Can you work these out from the model? Positions are in its coordinate system, mm. A direction names the side the tool comes from. Give positions to 0.01 mm unless a question says otherwise; leave off trailing zeros. Order: outer loops, then holes, each group sorted by start corner. A loop starts at its lowest first (then second) coordinate and runs counter-clockwise, first axis right, second up. Notation, with made-up numbers: M -17.5,66.25 L 29.5,66.25 A12 cw 29.5,73.25 Z; hole C 52.5,13 d11. An arc over 180 degrees is marked long. One line per question, with ' | ' between items. Start each with the question number.
1) For faces 1 (the flat face through (-17, 0, 39)), 2 (the flat face through (39.498, -13, 50)), 3 (the flat face through (28, -13, 61.81)), 4 (the flat face through (0, -13, 18)), which set-ups out of +Z, -Z, +X, -X, +Y, -Y let a thin tool reach every point of the face, with its end or its side?
2) Please list where these lines run through material, in increasing order: line 1 along Z through (x, y) = (37.5, -9.5); line 2 along Z through (x, y) = (69.5, -5) (3 decimals); line 3 along X through (y, z) = (-22, 63). Write a range as [from, to].
3) Thinking about a two-plate mould opening in X: for faces 5 (the flat face through (28, -13, 52.4)), 6 (the flat face through (39.498, -13, 69)), 7 (the flat face through (65, -13, 47.625)), 8 (the cylindrical face through (4.72, -12.52, 47.83)), which applies, +X half, -X half, draft (parallel to the pull), parting line (faces both ways), or undercut?
4) If we section it at B-B, the plane x = 47.5: Please give me the cut outline in (y, z) (3 decimals), plus the area to 3 significant figures.
5) If we section it at A-A, the plane z = 7.5: Please give me the cut outline in (x, y).
6) I'm going to push flat-ended pins straight in: pin 1 Ø1 at (x, y) = (-1.5, -21.5) entering from +Z; pin 2 Ø7 at (x, y) = (33.5, -16) entering from +Z; pin 3 Ø4.5 at (y, z) = (-9, 67) entering from -X; pin 4 Ø12 at (x, y) = (-12, -9.5) entering from -Z. Where does each tip first touch, or does it pass through?
```python
from build123d import *

# Parameters (mm, degrees)
F1_DEPTH = 25.4


with BuildPart() as f1:
    # F0 (on Front) → F1 (new body)
    with BuildSketch(Plane.XZ):
        Polygon((-82.55, 0), (0, 0), (0, 19.05), (-9.4102, 19.05), (-82.55, 19.05), align=None)
        with BuildLine():
            Line((-9.4102, 19.05), (0, 19.05))
            Line((0, 19.05), (0, 36.535349))
            ThreePointArc((0, 36.535349), (4.852166, 47.959566), (16.442551, 52.4002))
            Line((16.442551, 52.4002), (39.498304, 52.4002))
            Line((39.498304, 52.4002), (39.498304, 61.8104))
            Line((39.498304, 61.8104), (16.591319, 61.8104))
            ThreePointArc((16.591319, 61.8104), (14.455766, 61.780687), (12.330339, 61.570857))
            add(Edge.make_bspline(
                [(10.443617, 61.230316), (11.07103, 61.345589), (11.699943, 61.459099), (12.330339, 61.570857)],
                knots=[102.267957, 102.267957, 102.267957, 102.267957, 103.972602, 103.972602, 103.972602, 103.972602], degree=3))
            ThreePointArc((10.443617, 61.230316), (-3.83128, 52.37845), (-9.4102, 36.535349))
            Line((-9.4102, 36.535349), (-9.4102, 19.05))
        make_face()
        with BuildLine():
            add(Edge.make_bspline(
                [(-82.55, 19.05), (-59.439801, 41.052572), (-27.197229, 54.314634), (10.443617, 61.230316)],
                knots=[0, 0, 0, 0, 102.267957, 102.267957, 102.267957, 102.267957], degree=3))
            Line((-82.55, 19.05), (-9.4102, 19.05))
            Line((-9.4102, 19.05), (-9.4102, 36.535349))
            ThreePointArc((-9.4102, 36.535349), (-3.83128, 52.37845), (10.443617, 61.230316))
        make_face()
        with BuildLine():
            ThreePointArc((12.330339, 61.570857), (11.383749, 61.418475), (10.443617, 61.230316))
            add(Edge.make_bspline(
                [(10.443617, 61.230316), (11.07103, 61.345589), (11.699943, 61.459099), (12.330339, 61.570857)],
                knots=[102.267957, 102.267957, 102.267957, 102.267957, 103.972602, 103.972602, 103.972602, 103.972602], degree=3))
        make_face()
        Polygon((39.498304, 61.8104), (39.498304, 52.4002), (39.498304, 47.625), (90.298304, 47.625), (90.298304, 76.2), (39.498304, 76.2), align=None)
    extrude(amount=F1_DEPTH)


solid = f1.part
```
Results found:
1) face 1: +Z, -Z, +X, -X, +Y | face 2: -Z, +Y, -Y | face 3: +Z, -X, +Y, -Y | face 4: -Z, +X, +Y, -Y
2) line 1: z = [52.4, 61.81] | line 2: z = [47.625, 76.2] | line 3: x = [39.5, 90.3]
3) face 5: undercut | face 6: -X half | face 7: draft | face 8: undercut
4) outline: M -25.4,47.625 L 0,47.625 L 0,76.2 L -25.4,76.2 Z | area: 726 mm²
5) outline: M -82.55,-25.4 L 0,-25.4 L 0,0 L -82.55,0 Z
6) pin 1: stops at z = 58.89 | pin 2: stops at z = 61.81 | pin 3: stops at x = 39.5 | pin 4: stops at z = 0
